For this review, take the finished solid that the model builds, in its own axes (mm). Face numbers are marked on the shaded views. A direction names the side the tool comes from. Coordinates: 2 decimals unless noted, no trailing zeros. Order: outer loops, then holes, each group sorted by start corner. A loop starts at its lowest first (then second) coordinate and runs counter-clockwise, first axis right, second up. Notation, with made-up numbers: (64, 83.5) -> (90, 83.5) arc R13 cw to (90, 97.5) -> close; hole circle Ø6 at (-35.75, 46.25). An arc over 180 degrees is marked (long way). Write item = value, one per line. Start each with the question number.
1) Machinability: for the marked faces 1, 2 and 3, which of the approach directions +Z, -Z, +X, -X, +Y, -Y give a long, thin tool a straight path to every point of the face, cutting with its end or side? Answer none if there is none.
2) Insertion check: pin 1 Ø3.5 at (x, y) = (42.5, 0) entering from +Z; pin 2 Ø1 at (y, z) = (6, 25.5) entering from -X; pin 3 Ø10.5 at (x, y) = (42.5, 2) entering from +Z; pin 4 Ø1 at (x, z) = (-18.5, 46.5) entering from +Y. Each pin has a flat end and moves straight along its axis. Give the tip position at first contact, or say it passes through.
3) Draft analysis for pull direction X (two halves, no side actions). For the marked faces 4, 5 and 6, state which applies: +X half, -X half, draft (parallel to the pull), parting line (faces both ways), or undercut.
4) Consider section A-A on z = 25.5. Give the boundary of the cut face in (x, y).
5) Consider section D-D on z = 18. Give the boundary of the cut face in (x, y), and give its area (3 significant figures).
6) Consider section B-B on x = 42.5. Give the boundary of the cut face in (y, z).
7) Consider section C-C on z = 43. Give the boundary of the cut face in (x, y), and give its area (3 significant figures).
8) Wall thickness on probe 1 along Y at (x, z) = (42.5, 1.8); probe 2 along X at (y, z) = (-2, 29.5); probe 3 along Y at (x, z) = (20.5, 39.5): over which ranges is each line inside the solid? List them lowest first. Write a range as [from, to].
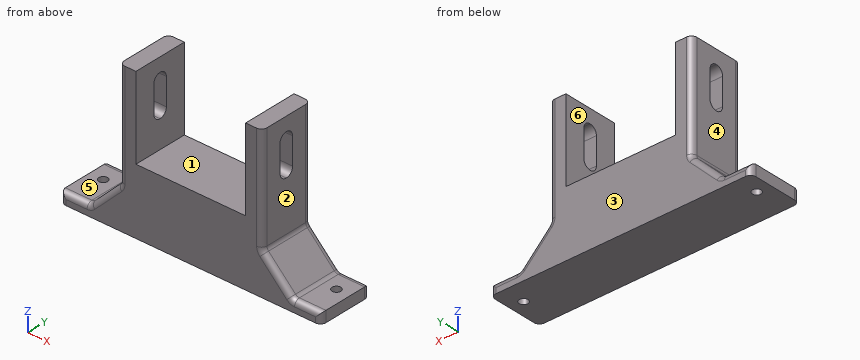
from build123d import *

# Parameters (mm, degrees)
F0_W     = 95
F0_H     = 20
F0_R     = 1.6
F1_DEPTH = 4
F3_DEPTH = 20
F4_SIZE  = 11
F6_DEPTH = 52
F7_F1_R  = 2
F7_F2_R  = 2


with BuildPart() as f1:
    # F0 (on Top) → F1 (new body)
    with BuildSketch(Plane.XY):
        with Locations((0, -2)):
            Rectangle(F0_W, F0_H)
        with Locations((-42.5, 0)):
            Circle(F0_R, mode=Mode.SUBTRACT)
        with Locations((42.5, 0)):
            Circle(F0_R, mode=Mode.SUBTRACT)
    extrude(amount=F1_DEPTH)

    # F2 (on face) → F3 (join, through all)
    with BuildSketch(Plane(origin=(0, 8, 0), x_dir=(-1, 0, 0), z_dir=(0, 1, 0))):
        Polygon((-26, 54), (-26, 4), (26, 4), (26, 54), (20, 54), (20, 24), (-20, 24), (-20, 54), align=None)
    extrude(amount=-F3_DEPTH)

    # F4
    f4_edges = [f1.edges().sort_by_distance(p)[0] for p in [
        (26, -2, 4),
        (-26, -2, 4),
    ]]
    chamfer(f4_edges, length=F4_SIZE)

    # F5 (on face) → F6 (cut, through all)
    with BuildSketch(Plane(origin=(-26, 0, 0), x_dir=(0, -1, 0), z_dir=(-1, 0, 0))):
        with BuildLine():
            ThreePointArc((2, 49), (0.1615223689, 48.2384776311), (-0.6, 46.4))
            Line((-0.6, 46.4), (-0.6, 36.6))
            ThreePointArc((-0.6, 36.6), (0.1615223689, 34.7615223689), (2, 34))
            ThreePointArc((2, 34), (3.8384776311, 34.7615223689), (4.6, 36.6))
            Line((4.6, 36.6), (4.6, 46.4))
            ThreePointArc((4.6, 46.4), (3.8384776311, 48.2384776311), (2, 49))
        make_face()
    extrude(amount=-F6_DEPTH, mode=Mode.SUBTRACT)

    # F7: fillet of radius 2 on 12 edges, made by hand

    # F7_f1
    f7_f1_edges = [f1.edges().sort_by_distance(p)[0] for p in [
        (37, -2, 4),
        (26, -2, 15),
        (-37, -2, 4),
        (-26, -2, 15),
    ]]
    fillet(f7_f1_edges, radius=F7_F1_R)

    # F7_f2
    f7_f2_edges = [f1.edges().sort_by_distance(p)[0] for p in [
        (31.5, 8, 9.5),
        (31.5, -12, 9.5),
        (-31.5, 8, 9.5),
        (-31.5, -12, 9.5),
        (-47.5, -12, 2),
        (-47.5, 8, 2),
        (47.5, -12, 2),
        (47.5, 8, 2),
        (-37.06306026, -12, 4.152240935),
        (-26.152240935, -12, 15.06306026),
        (-37.06306026, 8, 4.152240935),
        (-26.152240935, 8, 15.06306026),
        (37.06306026, -12, 4.152240935),
        (26.152240935, -12, 15.06306026),
        (37.06306026, 8, 4.152240935),
        (26.152240935, 8, 15.06306026),
    ]]
    fillet(f7_f2_edges, radius=F7_F2_R)


solid = f1.part
Answer sheet:
q1.face_1 = +Z, +Y, -Y
q1.face_2 = +Z, +X, +Y, -Y
q1.face_3 = +Z, -Z, +X, -X, +Y
q2.pin_1 = 4
q2.pin_2 = -26
q2.pin_3 = 4.09
q2.pin_4 = through
q3.face_4 = -X half
q3.face_5 = draft
q3.face_6 = undercut
q4.outline = (-26, -10) arc R2 ccw to (-24, -12) -> (-20, -12) -> (-20, 8) -> (-24, 8) arc R2 ccw to (-26, 6) -> close; (20, -12) -> (24, -12) arc R2 ccw to (26, -10) -> (26, 6) arc R2 ccw to (24, 8) -> (20, 8) -> close
q5.outline = (-26, -10) arc R2 ccw to (-24, -12) -> (24, -12) arc R2 ccw to (26, -10) -> (26, 6) arc R2 ccw to (24, 8) -> (-24, 8) arc R2 ccw to (-26, 6) -> close
q5.area = 1,040 mm2
q6.outline = (-12, 0) -> (-1.6, 0) -> (-1.6, 4) -> (-10, 4) arc R2 ccw to (-12, 2) -> close; (1.6, 0) -> (8, 0) -> (8, 2) arc R2 ccw to (6, 4) -> (1.6, 4) -> close
q7.outline = (-26, -10) arc R2 ccw to (-24, -12) -> (-20, -12) -> (-20, -4.6) -> (-26, -4.6) -> close; (-26, 0.6) -> (-20, 0.6) -> (-20, 8) -> (-24, 8) arc R2 ccw to (-26, 6) -> close; (20, -12) -> (24, -12) arc R2 ccw to (26, -10) -> (26, -4.6) -> (20, -4.6) -> close; (20, 0.6) -> (26, 0.6) -> (26, 6) arc R2 ccw to (24, 8) -> (20, 8) -> close
q7.area = 174 mm2
q8.probe_1 = [-12, -1.6], [1.6, 8]
q8.probe_2 = [-26, -20], [20, 26]
q8.probe_3 = [-12, -4.6], [0.6, 8]
